For this review, take the finished solid that the model builds, in its own axes (mm). A direction names the side the tool comes from. Round coordinates to 2 decimals unless told otherwise and drop trailing zeros. Loops run counter-clockwise (first coordinate to the right, second up) from the corner with the lowest first, then second, coordinate; pieces in that order, holes last. Notation, with made-up numbers: M -15.5,-3 L 41.5,-3 A10 cw 41.5,9 Z; hole C -13,-14.75 d9. An arc over 180 degrees is marked long. Write item = value, one per line. Start each with the question number.
```python
from build123d import *

# Parameters (mm, degrees)
BASE_EXTRUDE_DEPTH = 12.7
LPATTERN2_COUNT    = 2
LPATTERN2_PITCH    = 41.27246


with BuildPart() as part:
    # Sketch1 → Base-Extrude (new, symmetric)
    with BuildSketch(Plane.XY):
        with BuildLine():
            Line((17.6403, 16.339286512), (19.729882578, 19.063533504))
            ThreePointArc((19.729882578, 19.063533504), (19.156045845, 20.609744632), (17.6403, 21.2598))
            Line((17.6403, 21.2598), (14.70327367, 21.2598))
            ThreePointArc((14.70327367, 21.2598), (13.223883481, 20.647016519), (12.6111, 19.16762633))
            Line((12.6111, 19.16762633), (12.6111, 15.61465))
            Line((12.6111, 15.61465), (11.1125, 15.61465))
            Line((11.1125, 15.61465), (11.1125, 19.16762633))
            ThreePointArc((11.1125, 19.16762633), (12.164213258, 21.706686742), (14.70327367, 22.7584))
            Line((14.70327367, 22.7584), (17.6403, 22.7584))
            ThreePointArc((17.6403, 22.7584), (20.415434554, 21.446284653), (21.162428673, 18.4688666))
            Line((21.162428673, 18.4688666), (19.1389, 15.830735923))
            Line((19.1389, 15.830735923), (19.1389, 10.749129415))
            Line((19.1389, 10.749129415), (20.6375, 9.0662125))
            Line((20.6375, 9.0662125), (20.6375, -4.8244125))
            Line((20.6375, -4.8244125), (19.1389, -6.507329415))
            Line((19.1389, -6.507329415), (19.1389, -13.358784555))
            Line((19.1389, -13.358784555), (20.553458003, -14.773342558))
            ThreePointArc((20.553458003, -14.773342558), (18.729942105, -18.270236732), (15.019825564, -16.932883251))
            ThreePointArc((15.019825564, -16.932883251), (13.000752562, -16.523120627), (12.480559153, -18.5166))
            Line((12.480559153, -18.5166), (-12.480559153, -18.5166))
            ThreePointArc((-12.480559153, -18.5166), (-13.000752562, -16.523120627), (-15.019825564, -16.932883251))
            ThreePointArc((-15.019825564, -16.932883251), (-18.729942105, -18.270236732), (-20.553458003, -14.773342558))
            Line((-20.553458003, -14.773342558), (-19.1389, -13.358784555))
            Line((-19.1389, -13.358784555), (-19.1389, -6.507329415))
            Line((-19.1389, -6.507329415), (-20.6375, -4.8244125))
            Line((-20.6375, -4.8244125), (-20.6375, 9.0662125))
            Line((-20.6375, 9.0662125), (-19.1389, 10.749129415))
            Line((-19.1389, 10.749129415), (-19.1389, 15.830735923))
            Line((-19.1389, 15.830735923), (-21.162428673, 18.4688666))
            ThreePointArc((-21.162428673, 18.4688666), (-20.415434554, 21.446284653), (-17.6403, 22.7584))
            Line((-17.6403, 22.7584), (-14.70327367, 22.7584))
            ThreePointArc((-14.70327367, 22.7584), (-12.164213258, 21.706686742), (-11.1125, 19.16762633))
            Line((-11.1125, 19.16762633), (-11.1125, 15.61465))
            Line((-11.1125, 15.61465), (-12.6111, 15.61465))
            Line((-12.6111, 15.61465), (-12.6111, 19.16762633))
            ThreePointArc((-12.6111, 19.16762633), (-13.223883481, 20.647016519), (-14.70327367, 21.2598))
            Line((-14.70327367, 21.2598), (-17.6403, 21.2598))
            ThreePointArc((-17.6403, 21.2598), (-19.156045845, 20.609744632), (-19.729882578, 19.063533504))
            Line((-19.729882578, 19.063533504), (-17.6403, 16.339286512))
            Line((-17.6403, 16.339286512), (-17.6403, 10.17860201))
            Line((-17.6403, 10.17860201), (-19.1389, 8.495685095))
            Line((-19.1389, 8.495685095), (-19.1389, -4.253885095))
            Line((-19.1389, -4.253885095), (-17.6403, -5.93680201))
            Line((-17.6403, -5.93680201), (-17.6403, -13.979525))
            Line((-17.6403, -13.979525), (-19.1389, -15.478125))
            ThreePointArc((-19.1389, -15.478125), (-18.092238669, -16.906954381), (-16.414285827, -16.33992034))
            ThreePointArc((-16.414285827, -16.33992034), (-13.428073412, -14.819877156), (-10.898992189, -17.018))
            Line((-10.898992189, -17.018), (10.898992189, -17.018))
            ThreePointArc((10.898992189, -17.018), (13.323359075, -14.834630878), (16.30518861, -16.15877141))
            ThreePointArc((16.30518861, -16.15877141), (17.990302879, -16.935279743), (19.1389, -15.478125))
            Line((19.1389, -15.478125), (17.6403, -13.979525))
            Line((17.6403, -13.979525), (17.6403, -5.93680201))
            Line((17.6403, -5.93680201), (19.1389, -4.253885095))
            Line((19.1389, -4.253885095), (19.1389, 8.495685095))
            Line((19.1389, 8.495685095), (17.6403, 10.17860201))
            Line((17.6403, 10.17860201), (17.6403, 16.339286512))
        make_face()
    base_extrude = extrude(amount=BASE_EXTRUDE_DEPTH, both=True)

    # LPattern2: Base-Extrude ×2
    with Locations(*[(i * LPATTERN2_PITCH, 0, 0) for i in range(1, LPATTERN2_COUNT)]):
        add(base_extrude)


solid = part.part
```
(1) Draft analysis for pull direction X (two halves, no side actions). For faces 4 (the flat face through (-19.899, 9.896, 0.178)), 5 (the flat face through (-12.611, 17, 0)), 6 (the cylindrical face through (62, 21, 0)), state which applies: +X half, -X half, draft (parallel to the pull), parting line (faces both ways), or undercut.
(2) Add section B-B on y = 1. Write out the cut boundary in (x, z), and give its area (3 significant figures).
(3) For pin 1 Ø4 at (x, z) = (31, 0.5) entering from +Y; pin 2 Ø10 at (x, z) = (-3, 7) entering from +Y; pin 3 Ø1.5 at (y, z) = (-10.5, 4.5) entering from -X; pin 4 Ø4 at (x, y) = (16.5, -2) entering from -Z, all flat-tipped, find the tip position at first contact; note any pin that passes through.
(4) Add section A-A on y = -7.5. Write out the cut boundary in (x, z).
(5) Add section D-D on z = -0.75. Count the separate pieces of the cut face and the enclosed holes in it, and give its area (3 significant figures).
(6) Tool access review of faces 1 (the flat face through (-19.878, -5.678, 0.178)), 2 (the flat face through (59.65, -5.11, 0.18)), 3 (the flat face through (57, 22.758, 0)): name each direction out of +Z, -Z, +X, -X, +Y, -Y from which nothing blocks a thin tool from reaching the whole face with its end or side.
(7) Wall thickness on L1, parallel to X at y = 2, z = -6.5; L2, parallel to X at y = 12, z = -5; L3, parallel to X at y = 9, z = -2: over which ranges is each line inside the solid? List them lowest first.
(8) Add section C-C on x = 37.5. Write out the cut boundary in (y, z).
Answer sheet:
q1.face_4 = -X half
q1.face_5 = undercut
q1.face_6 = +X half
q2.outline = M -20.64,-12.7 L -19.14,-12.7 L -19.14,12.7 L -20.64,12.7 Z; M 19.14,-12.7 L 22.13,-12.7 L 22.13,12.7 L 19.14,12.7 Z; M 60.41,-12.7 L 61.91,-12.7 L 61.91,12.7 L 60.41,12.7 Z
q2.area = 152 mm²
q3.pin_1 = 21.81
q3.pin_2 = -17.02
q3.pin_3 = -19.14
q3.pin_4 = through
q4.outline = M -19.14,-12.7 L -17.64,-12.7 L -17.64,12.7 L -19.14,12.7 Z; M 17.64,-12.7 L 19.14,-12.7 L 19.14,12.7 L 17.64,12.7 Z; M 22.13,-12.7 L 23.63,-12.7 L 23.63,12.7 L 22.13,12.7 Z; M 58.91,-12.7 L 60.41,-12.7 L 60.41,12.7 L 58.91,12.7 Z
q5.separate_pieces = 1
q5.enclosed_holes = 2
q5.area = 451 mm²
q6.face_1 = +Z, -Z, -X
q6.face_2 = +Z, -Z
q6.face_3 = +Z, -Z, +X, -X, +Y
q7.L1 = -20.64 to -19.14, 19.14 to 22.13, 60.41 to 61.91
q7.L2 = -19.14 to -17.64, 17.64 to 19.14, 22.13 to 23.63, 58.91 to 60.41
q7.L3 = -20.64 to -18.69, 18.69 to 22.58, 59.96 to 61.91
q8.outline = M -18.52,-12.7 L -17.02,-12.7 L -17.02,12.7 L -18.52,12.7 Z
